from build123d import *

# Parameters (mm, degrees)
IZIM1_R                     = 50
Y_KSEKLIK_EKSTR_ZYON1_DEPTH = 100
Y_KSEKLIK_EKSTR_ZYON2_REACH = 202
IZIM3_R                     = 45


with BuildPart() as part:
    # Çizim1 → Yükseklik-Ekstrüzyon1 (new body)
    with BuildSketch(Plane.XY):
        with BuildLine():
            Line((-80, -40), (-80, 40))
            Line((-80, 40), (-22.281665693, 61.061668614))
            ThreePointArc((-22.281665693, 61.061668614), (65, 0), (-22.281665693, -61.061668614))
            Line((-22.281665693, -61.061668614), (-80, -40))
        make_face()
        Circle(IZIM1_R, mode=Mode.SUBTRACT)
    extrude(amount=Y_KSEKLIK_EKSTR_ZYON1_DEPTH)

    # Çizim3 → Yükseklik-Ekstrüzyon2 (add, up to next)
    with BuildSketch(Plane(origin=(120, 0, 0), x_dir=(0, 0, -1), z_dir=(1, 0, 0)), mode=Mode.PRIVATE) as y_kseklik_ekstr_zyon2_sk1:
        with Locations((-50, 0)):
            Circle(IZIM3_R)
    y_kseklik_ekstr_zyon2_tool1 = extrude(y_kseklik_ekstr_zyon2_sk1.sketch, amount=-Y_KSEKLIK_EKSTR_ZYON2_REACH, mode=Mode.PRIVATE) - part.part
    add(y_kseklik_ekstr_zyon2_tool1.solids().sort_by_distance((120, 0, 50))[0])

    # Çizim6 → Döndür1 (revolve)
    with BuildSketch(Plane.XY.offset(50)):
        Polygon((120, 0), (120, -20), (134, -20), (134, -25), (149, -25), (149, -14.033097), (158.403875038, -10.632048004), (158.403875038, -5.4519389), (195, 0), align=None)
    revolve(axis=Axis((-133.942981773, 0, 50), (1, 0, 0)))


solid = part.part
Geometry: final body of the model. Coordinates: model frame, mm. A direction names the side the tool comes from. Give positions to 0.01 mm unless a question says otherwise; leave off trailing zeros. Order: outer loops, then holes, each group sorted by start corner. A loop starts at its lowest first (then second) coordinate and runs counter-clockwise, first axis right, second up. Notation, with made-up numbers: (12, -33.75) -> (55, -33.75) arc R7 ccw to (55, -26.75) -> close; hole circle Ø4 at (20, -5). An arc over 180 degrees is marked (long way). Put each result on its own line as item: value.
Q1. Draft query along X for faces 1 (the face through (41.39, 50.12, 49.3)), 2 (the face through (47.69, 15.02, 49.3)), 3 (the face through (158.404, 5, 47)). Return one class per face: released by +X, released by -X, zero draft, split by the parting line, or undercut.
Here are the results:
face 1: split by the parting line
face 2: undercut
face 3: released by +X
Q2. Pin query (flat end, axial travel): pin 1 (10 mm diameter, centred on x = 7.5, y = -43, fed in from +Z) (3 decimals); pin 2 (4 mm diameter, centred on x = 104.5, y = 39.5, fed in from +Z); pin 3 (1 mm diameter, centred on x = 69, z = 42, fed in from -Y); pin 4 (1.5 mm diameter, centred on x = 62.5, z = 63, fed in from -Y). Return the tip coordinate at first contact, or that it passes through.
Here are the results:
pin 1: passes through
pin 2: stops at z = 74.87
pin 3: stops at y = -44.37
pin 4: stops at y = -43.3
Q3. Section C-C, the plane y = 28. Return loops of the section in (x, z), then the cut area to 3 significant figures.
Here are the results:
outline: (-80, 0) -> (-41.42, 0) -> (-41.42, 100) -> (-80, 100) -> close; (41.42, 0) -> (58.66, 0) -> (58.66, 14.77) -> (120, 14.77) -> (120, 85.23) -> (58.66, 85.23) -> (58.66, 100) -> (41.42, 100) -> close
area: 9,900 mm^2
Q4. Section A-A, the plane x = 0. Return loops of the section in (y, z), then the cut area to 3 significant figures.
Here are the results:
outline: (-65, 0) -> (-50, 0) -> (-50, 100) -> (-65, 100) -> close; (50, 0) -> (65, 0) -> (65, 100) -> (50, 100) -> close
area: 3,000 mm^2
Q5. Section B-B, the plane z = 20. Return loops of the section in (x, y), then the cut area to 3 significant figures.
Here are the results:
outline: (-80, -40) -> (-22.28, -61.06) arc R65 ccw to (55.68, -33.54) -> (120, -33.54) -> (120, 33.54) -> (55.68, 33.54) arc R65 ccw to (-22.28, 61.06) -> (-80, 40) -> close; hole circle Ø100 at (0, 0)
area: 11,300 mm^2
Q6. Section D-D, the plane x = 116.5. Return loops of the section in (y, z).
Here are the results:
outline: circle Ø90 at (0, 50)
Q7. Reachability of faces 4 (the face through (-51.5, 50.4, 49.3)), 5 (the face through (134, -11, 33)), 6 (the face through (149, -11, 61)) from +Z, -Z, +X, -X, +Y, -Y: full face, straight path, thin tool, end or side. Return the list, or none.
Here are the results:
face 4: +Z, -Z, -X, +Y
face 5: none
face 6: +X
Q8. Material intervals for L1, parallel to Y at x = 0, z = 72; L2, parallel to X at y = 37, z = 17.5; L3, parallel to X at y = -27, z = 7, sorted ascending.
Here are the results:
L1: y = -65 to -50, 50 to 65
L2: x = -80 to -33.63, 33.63 to 53.44
L3: x = -80 to -42.08, 42.08 to 59.13
